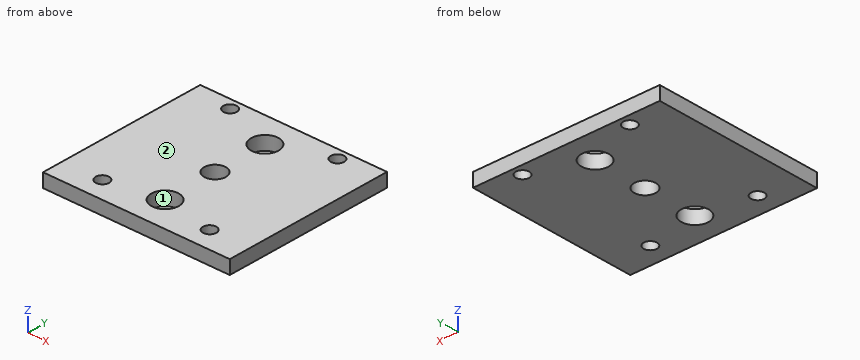
from build123d import *

# Parameters (mm, degrees)
CROQUIS1_W              = 87
CROQUIS1_H              = 80
CROQUIS1_R              = 3.1
CROQUIS1_R_2            = 6.35
CROQUIS1_R_3            = 5
SALIENTE_EXTRUIR1_DEPTH = 6.35


with BuildPart() as part:
    # Croquis1 → Saliente-Extruir1 (new body)
    with BuildSketch(Plane.XY):
        Rectangle(CROQUIS1_W, CROQUIS1_H)
        with Locations((-25, 35)):
            Circle(CROQUIS1_R, mode=Mode.SUBTRACT)
        with Locations((25, 35)):
            Circle(CROQUIS1_R, mode=Mode.SUBTRACT)
        with Locations((0, 25.4)):
            Circle(CROQUIS1_R_2, mode=Mode.SUBTRACT)
        with Locations((0, -25.4)):
            Circle(CROQUIS1_R_2, mode=Mode.SUBTRACT)
        with Locations((-25, -30)):
            Circle(CROQUIS1_R, mode=Mode.SUBTRACT)
        with Locations((25, -30)):
            Circle(CROQUIS1_R, mode=Mode.SUBTRACT)
        Circle(CROQUIS1_R_3, mode=Mode.SUBTRACT)
    extrude(amount=SALIENTE_EXTRUIR1_DEPTH)


solid = part.part
Work out the finished part from the listing and answer in its coordinate system (mm). Face numbers are marked on the shaded views. Round coordinates to 2 decimals unless told otherwise and drop trailing zeros. Loops run counter-clockwise (first coordinate to the right, second up) from the corner with the lowest first, then second, coordinate; pieces in that order, holes last. Notation, with made-up numbers: (72, 66) - (84, 66) arc R13 ccw to (84, 72) - close; hole circle Ø5 at (20, 44). An arc over 180 degrees is marked (long way). Use one line per item in the form item = value. Start each with the question number.
(1) Find section D-D on x = 25. Determine the outline of the cut face in (y, z).
(2) A flat-ended cylindrical pin translates along its axis: P1, Ø7.5, axis at x = 0, y = -25.4, coming from the -Z side. Find the tip coordinate at first contact, or state that the pin passes through.
(3) Determine the mould class of the marked faces 1 and 2 for opening direction X: +X half, -X half, draft (parallel to the pull), parting line (faces both ways), or undercut.
(4) Consider line 1 (Y direction, x = -25, z = 1.75); line 2 (Y direction, x = 0, z = 3.75); line 3 (X direction, y = 33.5, z = 2.5). Determine where each line is inside the solid, lowest interval first.
(5) Find section A-A on y = 35. Determine the outline of the cut face in (x, z), and give its area (3 significant figures).
(6) Find section C-C on y = 0. Determine the outline of the cut face in (x, z).
(7) Find section B-B on z = 5.25. Determine the outline of the cut face in (x, y), and give its area (3 significant figures).
Answer list:
q1.outline = (-40, 0) - (-33.1, 0) - (-33.1, 6.35) - (-40, 6.35) - close; (-26.9, 0) - (31.9, 0) - (31.9, 6.35) - (-26.9, 6.35) - close; (38.1, 0) - (40, 0) - (40, 6.35) - (38.1, 6.35) - close
q2.P1 = through
q3.face_1 = undercut
q3.face_2 = draft
q4.line_1 = -40 to -33.1, -26.9 to 31.9, 38.1 to 40
q4.line_2 = -40 to -31.75, -19.05 to -5, 5 to 19.05, 31.75 to 40
q4.line_3 = -43.5 to -27.71, -22.29 to 22.29, 27.71 to 43.5
q5.outline = (-43.5, 0) - (-28.1, 0) - (-28.1, 6.35) - (-43.5, 6.35) - close; (-21.9, 0) - (21.9, 0) - (21.9, 6.35) - (-21.9, 6.35) - close; (28.1, 0) - (43.5, 0) - (43.5, 6.35) - (28.1, 6.35) - close
q5.area = 474 mm^2
q6.outline = (-43.5, 0) - (-5, 0) - (-5, 6.35) - (-43.5, 6.35) - close; (5, 0) - (43.5, 0) - (43.5, 6.35) - (5, 6.35) - close
q7.outline = (-43.5, -40) - (43.5, -40) - (43.5, 40) - (-43.5, 40) - close; hole circle Ø6.2 at (-25, -30); hole circle Ø6.2 at (-25, 35); hole circle Ø12.7 at (0, -25.4); hole circle Ø12.7 at (0, 25.4); hole circle Ø10 at (0, 0); hole circle Ø6.2 at (25, -30); hole circle Ø6.2 at (25, 35)
q7.area = 6,510 mm^2
